```python
from build123d import *

# Parameters (mm, degrees)
SKETCH1_R           = 20
BOSS_EXTRUDE1_DEPTH = 10
SKETCH2_W           = 40
SKETCH2_H           = 5
BOSS_EXTRUDE2_DEPTH = 10
SKETCH3_R           = 15.875
CUT_EXTRUDE1_DEPTH  = 31


with BuildPart() as part:
    # Sketch1 → Boss-Extrude1 (new body)
    with BuildSketch(Plane.XY):
        Circle(SKETCH1_R)
    extrude(amount=BOSS_EXTRUDE1_DEPTH)

    # Sketch2 → Boss-Extrude2 (add)
    with BuildSketch(Plane(origin=(0, 0, 0), x_dir=(-1, 0, 0), z_dir=(0, 0, -1))):
        with Locations((0, -17.5)):
            Rectangle(SKETCH2_W, SKETCH2_H)
    extrude(amount=-BOSS_EXTRUDE2_DEPTH)

    # Sketch3 → Cut-Extrude1 (cut, through all)
    with BuildSketch(Plane(origin=(0, 0, 0), x_dir=(-1, 0, 0), z_dir=(0, 0, -1))):
        Circle(SKETCH3_R)
    extrude(amount=-CUT_EXTRUDE1_DEPTH, mode=Mode.SUBTRACT)


solid = part.part
```
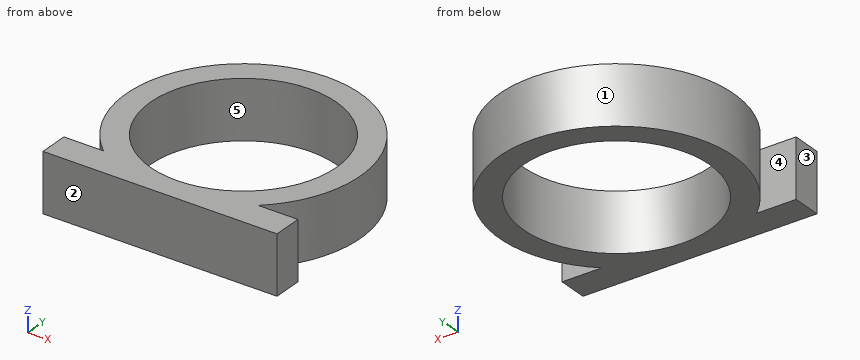
Can you work these out from the model? Positions are in its coordinate system, mm. Face numbers are marked on the shaded views. A direction names the side the tool comes from. Coordinates: 2 decimals unless noted, no trailing zeros. Loops run counter-clockwise (first coordinate to the right, second up) from the corner with the lowest first, then second, coordinate; pieces in that order, holes last. Notation, with made-up numbers: (28, -33.75) -> (49, -33.75) arc R32 ccw to (49, 0.25) -> close; hole circle Ø7 at (-2, 20). An arc over 180 degrees is marked (long way). Put each result on its own line as item: value. Start each with the question number.
Q1. I'm going to push flat-ended pins straight in: P1, Ø1.5, axis at y = 4, z = 7, coming from the +X side; P2, Ø10, axis at x = -9, y = -3, coming from the -Z side; P3, Ø2, axis at y = 12.5, z = 2, coming from the -X side. Where does each tip first touch, or does it pass through?
Q2. I want a section at A-A (y = 0). Write out the boundary of the cut face in (x, z) (3 decimals).
Q3. If I drill on line 1 (Y direction, x = 0, z = 3) (3 decimals); line 2 (X direction, y = 0.5, z = 8.25); line 3 (Y direction, x = 3.5, z = 5.75), over which ranges is the centre line in solid material (lowest first)? Write a range as [from, to].
Q4. I want a section at D-D (x = -15). Write out the boundary of the cut face in (y, z), plus the area to 3 significant figures.
Q5. For the marked faces 4 and 5, which set-ups out of +Z, -Z, +X, -X, +Y, -Y let a thin tool reach every point of the face, with its end or its side?
Q6. Thinking about a two-plate mould opening in Y: for the marked faces 1, 2 and 3, which applies, pulls with the +Y half, pulls with the -Y half, needs draft (parallel to the pull), parting line crosses it, or undercut?
Q7. I want a section at C-C (z = 3.75). Write out the boundary of the cut face in (x, y) (3 decimals), plus the area to 3 significant figures.
Taken from the geometry:
1. P1: stops at x = 19.73
1. P2: passes through
1. P3: stops at x = -16.36
2. outline: (-20, 0) -> (-15.875, 0) -> (-15.875, 10) -> (-20, 10) -> close; (15.875, 0) -> (20, 0) -> (20, 10) -> (15.875, 10) -> close
3. line 1: y = [-20, -15.875], [15.875, 20]
3. line 2: x = [-19.99, -15.87], [15.87, 19.99]
3. line 3: y = [-20, -15.48], [15.48, 19.69]
4. outline: (-20, 0) -> (-15, 0) -> (-15, 10) -> (-20, 10) -> close; (-13.23, 0) -> (-5.2, 0) -> (-5.2, 10) -> (-13.23, 10) -> close; (5.2, 0) -> (13.23, 0) -> (13.23, 10) -> (5.2, 10) -> close
4. area: 211 mm2
5. face 4: +Z, -Z, -X
5. face 5: +Z, -Z
6. face 1: undercut
6. face 2: pulls with the -Y half
6. face 3: needs draft
7. outline: (-20, -20) -> (20, -20) -> (20, -15) -> (13.229, -15) arc R20 ccw (long way) to (-13.229, -15) -> (-20, -15) -> close; hole circle Ø31.75 at (0, 0)
7. area: 574 mm2
